The model under review builds one solid part; all positions refer to its coordinate system, in mm. Face numbers are marked on the shaded views. A direction names the side the tool comes from. Give positions to 0.01 mm unless a question says otherwise; leave off trailing zeros. Order: outer loops, then holes, each group sorted by start corner. A loop starts at its lowest first (then second) coordinate and runs counter-clockwise, first axis right, second up. Notation, with made-up numbers: (87.25, -27) -> (109.25, -27) arc R11 cw to (109.25, -11) -> close; hole circle Ø10 at (7, 6). An arc over 180 degrees is marked (long way). Use one line per item in the form item = value.
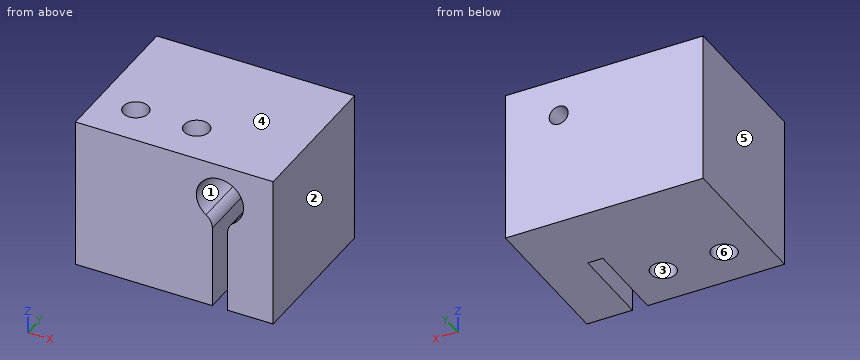
```python
from build123d import *

# Parameters (mm, degrees)
SKETCH_1_W          = 26
SKETCH_1_H          = 20
EXTRUDE_1_DEPTH     = 25
CUT_EXTRUDE_1_DEPTH = 16
FILLET_1_R          = 2
SKETCH_3_R          = 1.25
CUT_EXTRUDE_2_DEPTH = 23.912878475
SKETCH_4_R          = 1.65
CUT_EXTRUDE_3_DEPTH = 35.554305086
SKETCH_5_W          = 20
SKETCH_5_H          = 5
CUT_EXTRUDE_4_DEPTH = 38.429934544


with BuildPart() as part:
    # 草图1 → 凸台-拉伸1 (new body)
    with BuildSketch(Plane(origin=(0, 0, 0), x_dir=(1, 0, 0), z_dir=(0, 1, 0))):
        Rectangle(SKETCH_1_W, SKETCH_1_H)
    extrude(amount=EXTRUDE_1_DEPTH)

    # 草图2 → 切除-拉伸1 (cut)
    with BuildSketch(Plane.XZ):
        with BuildLine():
            Line((5, 2.06571985), (5, -10))
            Line((5, -10), (7, -10))
            Line((7, -10), (7, 2.06571985))
            ThreePointArc((7, 2.06571985), (6, 8.1), (5, 2.06571985))
        make_face()
    extrude(amount=-CUT_EXTRUDE_1_DEPTH, mode=Mode.SUBTRACT)

    # 圆角1
    fillet_1_edges = [part.edges().sort_by_distance(p)[0] for p in [
        (5, 8, 2.06571985),
        (7, 8, 2.06571985),
    ]]
    fillet(fillet_1_edges, radius=FILLET_1_R)

    # 草图3 → 切除-拉伸2 (cut, through all)
    with BuildSketch(Plane.XZ.offset(-16)):
        with Locations(Location((6, 5, 0), (0, 0, 270))):
            Circle(SKETCH_3_R)
    extrude(amount=-CUT_EXTRUDE_2_DEPTH, mode=Mode.SUBTRACT)

    # 草图4 → 切除-拉伸3 (cut, through all)
    with BuildSketch(Plane(origin=(0, 0, -10), x_dir=(-1, 0, 0), z_dir=(0, 0, -1))):
        with Locations((8, 10.5)):
            Circle(SKETCH_4_R)
        with Locations((0, 10.5)):
            Circle(SKETCH_4_R)
    extrude(amount=-CUT_EXTRUDE_3_DEPTH, mode=Mode.SUBTRACT)

    # 草图5 → 切除-拉伸4 (cut, through all)
    with BuildSketch(Plane(origin=(13, 0, 0), x_dir=(0, 0, -1), z_dir=(1, 0, 0))):
        with Locations((0, 2.5)):
            Rectangle(SKETCH_5_W, SKETCH_5_H)
    extrude(amount=-CUT_EXTRUDE_4_DEPTH, mode=Mode.SUBTRACT)


solid = part.part
```
1. Add section B-B on x = 0. Give the boundary of the cut face in (y, z).
Values:
outline = (5, -10) -> (8.85, -10) -> (8.85, 10) -> (5, 10) -> close; (12.15, -10) -> (25, -10) -> (25, 10) -> (12.15, 10) -> close
2. For pin 1 Ø3 at (x, y) = (0, 10.5) entering from +Z, flat-tipped, find the tip position at first contact; note if it passes through.
Values:
pin_1 = through
3. Add section A-A on z = 5. Give the boundary of the cut face in (x, y), then the cut area to 3 significant figures.
Values:
outline = (-13, 5) -> (2.9, 5) -> (2.9, 16) -> (4.75, 16) -> (4.75, 25) -> (-13, 25) -> close; (7.25, 16) -> (9.1, 16) -> (9.1, 5) -> (13, 5) -> (13, 25) -> (7.25, 25) -> close; hole circle Ø3.3 at (-8, 10.5); hole circle Ø3.3 at (0, 10.5)
area = 412 mm^2
4. Add section D-D on y = 13. Give the boundary of the cut face in (x, z), then the cut area to 3 significant figures.
Values:
outline = (-13, -10) -> (5, -10) -> (5, 0.88) arc R2 ccw to (4.18, 2.49) arc R3.1 cw (long way) to (7.82, 2.49) arc R2 ccw to (7, 0.88) -> (7, -10) -> (13, -10) -> (13, 10) -> (-13, 10) -> close
area = 465 mm^2
5. Add section C-C on z = -7.75. Give the boundary of the cut face in (x, y), then the cut area to 3 significant figures.
Values:
outline = (-13, 5) -> (5, 5) -> (5, 16) -> (7, 16) -> (7, 5) -> (13, 5) -> (13, 25) -> (-13, 25) -> close; hole circle Ø3.3 at (-8, 10.5); hole circle Ø3.3 at (0, 10.5)
area = 481 mm^2
6. Tool access review of the marked faces 1 and 2: name each direction out of +Z, -Z, +X, -X, +Y, -Y from which nothing blocks a thin tool from reaching the whole face with its end or side.
Values:
face_1 = -Y
face_2 = +Z, -Z, +X, +Y, -Y
7. The part is to be moulded in two halves that separate along X. For the marked faces 3, 4, 5 and 6, say which applies: +X half, -X half, draft (parallel to the pull), parting line (faces both ways), or undercut.
Values:
face_3 = undercut
face_4 = draft
face_5 = -X half
face_6 = undercut
8. For L1, parallel to Y at x = -8, z = -2; L2, parallel to X at y = 9, z = -5; L3, parallel to X at y = 19, z = 5, list the stretches that pass through material, from the lowest coordinate up.
Values:
L1 = 5 to 8.85, 12.15 to 25
L2 = -13 to -8.69, -7.31 to -0.69, 0.69 to 5, 7 to 13
L3 = -13 to 4.75, 7.25 to 13
